Here's the drawing with two shaded views (mm, measured from the low corner). I have some questions. Coordinates: 2 decimals unless noted, no trailing zeros. Order: outer loops, then holes, each group sorted by start corner. A loop starts at its lowest first (then second) coordinate and runs counter-clockwise, first axis right, second up. Notation, with made-up numbers: (-14.75, -20.75) -> (41.25, -20.75) arc R23 ccw to (41.25, -7.75) -> close; hole circle Ø2 at (-25, 51.25). An arc over 180 degrees is marked (long way). Answer as a JSON object with one key per item and string values. Group by question number.
(1) I want a section at B-B, the plane y = 5.5. List the corners of the cut face in (x, z) for me, plus the area to 3 significant figures.
(2) I want a section at D-D, the plane z = 18. List the corners of the cut face in (x, y) for me, plus the area to 3 significant figures.
(3) I want a section at C-C, the plane z = 7. List the corners of the cut face in (x, y) for me.
(4) If we mould it in two halves opening along Y, with no side actions, what happens to the marked faces 1 and 2? For each: pulls with the +Y half, pulls with the -Y half, needs draft (parallel to the pull), parting line crosses it, or undercut.
(5) I need wall thicknesses on line 1 (Z direction, x = 5.5, y = 10.75); line 2 (Y direction, x = 5.75, z = 37); line 3 (Y direction, x = 8, z = 35). Which ranges of each line are inside material? Lowest first, please.
(6) For pin 1 (2 mm diameter, centred on y = 1.5, z = 36.5, fed in from -X); pin 2 (1.5 mm diameter, centred on x = 3, y = 3, fed in from -Z); pin 3 (1 mm diameter, centred on x = 7, z = 33.5, fed in from -Y), each with a flat end and sliding along its axis, tell me the tip position at first contact or that it passes through.
(7) I want a section at A-A, the plane x = 5.5. List the corners of the cut face in (y, z) for me.
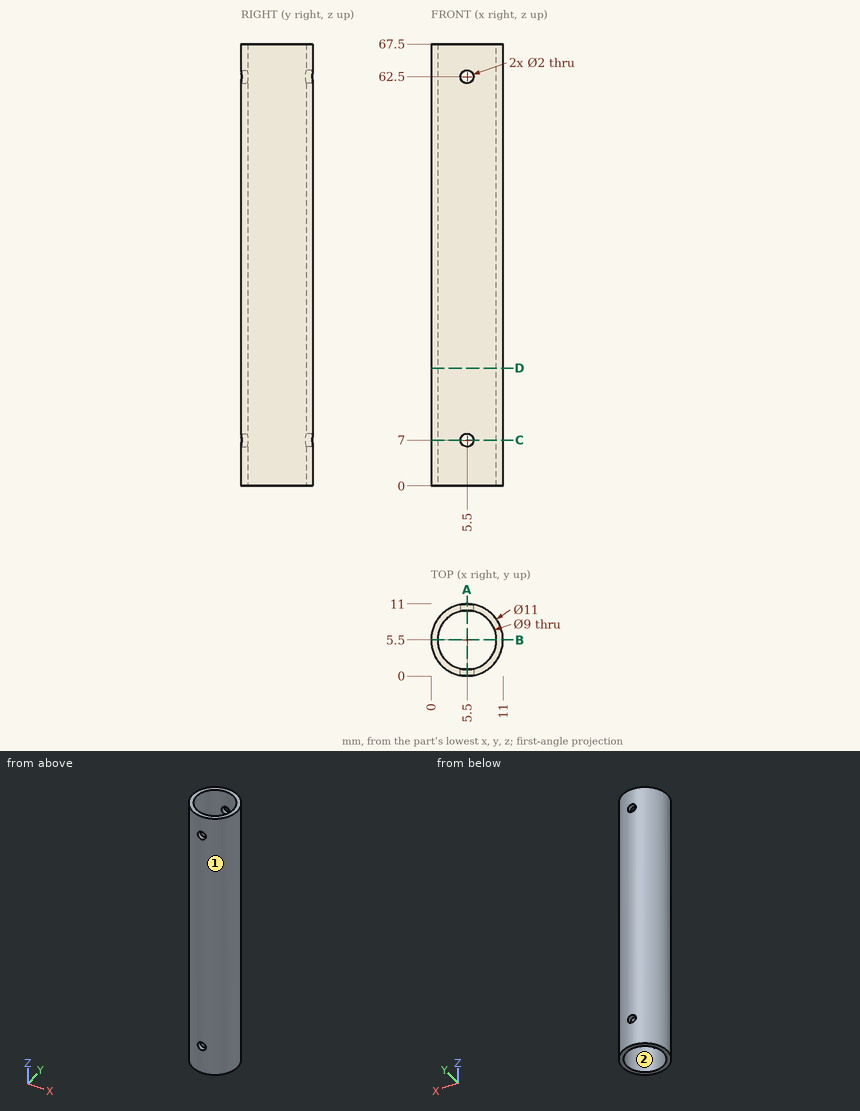
Computed values:
{
 "1": {"outline": "(0, 0) -> (1, 0) -> (1, 67.5) -> (0, 67.5) -> close; (10, 0) -> (11, 0) -> (11, 67.5) -> (10, 67.5) -> close", "area": "135 mm2"},
 "2": {"outline": "circle Ø11 at (5.5, 5.5); hole circle Ø9 at (5.5, 5.5)", "area": "31.4 mm2"},
 "3": {"outline": "(4.5, 0.09) -> (4.5, 1.11) arc R4.5 cw to (4.5, 9.89) -> (4.5, 10.91) arc R5.5 ccw to start; (6.5, 0.09) arc R5.5 ccw to (6.5, 10.91) -> (6.5, 9.89) arc R4.5 cw to (6.5, 1.11) -> close"},
 "4": {"face 1": "parting line crosses it", "face 2": "undercut"},
 "5": {"line 1": "z = 0 to 6, 8 to 61.5, 63.5 to 67.5", "line 2": "y = 0.01 to 1.01, 9.99 to 10.99", "line 3": "y = 0.6 to 1.76, 9.24 to 10.4"},
 "6": {"pin 1": "stops at x = 0.89", "pin 2": "passes through", "pin 3": "stops at y = 0.09"},
 "7": {"outline": "(0, 0) -> (1, 0) -> (1, 6) -> (0, 6) -> close; (0, 8) -> (1, 8) -> (1, 61.5) -> (0, 61.5) -> close; (0, 63.5) -> (1, 63.5) -> (1, 67.5) -> (0, 67.5) -> close; (10, 0) -> (11, 0) -> (11, 6) -> (10, 6) -> close; (10, 8) -> (11, 8) -> (11, 61.5) -> (10, 61.5) -> close; (10, 63.5) -> (11, 63.5) -> (11, 67.5) -> (10, 67.5) -> close"}
}
